Could you check a few things on this model? Use its own coordinates, in mm. Round coordinates to 2 decimals unless told otherwise and drop trailing zeros. Write each loop counter-clockwise with the first axis right and the second up, starting at its lowest first coordinate (ties: lowest second). Pieces come first, ordered by that corner, then holes. Notation, with made-up numbers: (-5.5, 1.25) -> (39.5, 1.25) arc R16 ccw to (39.5, 31.25) -> close; hole circle Ø1 at (4.5, 38.5). An arc over 180 degrees is marked (long way). Answer in a Markdown table with one row per item.
from build123d import *

# Parameters (mm, degrees)
SKETCH2_W           = 18.6
SKETCH2_H           = 76.6
SKETCH2_R           = 3.75
BOSS_EXTRUDE1_DEPTH = 1


with BuildPart() as part:
    # Sketch2 → Boss-Extrude1 (new body)
    with BuildSketch(Plane(origin=(0, 0, 0), x_dir=(1, 0, 0), z_dir=(0, 1, 0))):
        with Locations((-31.729014151, 24.017653569)):
            Rectangle(SKETCH2_W, SKETCH2_H)
        with Locations((-34.229014151, 53.517653569)):
            Circle(SKETCH2_R, mode=Mode.SUBTRACT)
    extrude(amount=BOSS_EXTRUDE1_DEPTH)


solid = part.part
1) Please list where these lines run through material, in increasing order: line 1 (Z direction, x = -37.5, y = 0.3); line 2 (Z direction, x = -31, y = 0.45); line 3 (X direction, y = 0.55, z = -55).
Findings:
| item | result |
|---|---|
| line 1 | z = -62.32 to -55.35, -51.68 to 14.28 |
| line 2 | z = -62.32 to -55.42, -51.61 to 14.28 |
| line 3 | x = -41.03 to -37.67, -30.78 to -22.43 |
2) Imagine slicing it at B-B, the plane y = 0.8. Please give me the cut outline in (x, z).
Findings:
| item | result |
|---|---|
| outline | (-41.03, -62.32) -> (-22.43, -62.32) -> (-22.43, 14.28) -> (-41.03, 14.28) -> close; hole circle Ø7.5 at (-34.23, -53.52) |
3) Imagine slicing it at A-A, the plane x = -36. Please give me the cut outline in (y, z), plus the area to 3 significant figures.
Findings:
| item | result |
|---|---|
| outline | (0, -62.32) -> (1, -62.32) -> (1, -56.82) -> (0, -56.82) -> close; (0, -50.21) -> (1, -50.21) -> (1, 14.28) -> (0, 14.28) -> close |
| area | 70.0 mm^2 |
4) Thinking about a two-plate mould opening in X: for faces 1 (the face through (-32, 1, -25)), 2 (the face through (-30.65, 0.49, -54.64)), which applies, +X half, -X half, draft (parallel to the pull), parting line (faces both ways), or undercut?
Findings:
| item | result |
|---|---|
| face 1 | draft |
| face 2 | undercut |
